The listing builds one solid part. Answer for the finished solid, in the listing's coordinates (mm). Face numbers are marked on the shaded views. A direction names the side the tool comes from. Coordinates: 2 decimals unless noted, no trailing zeros. Loops run counter-clockwise (first coordinate to the right, second up) from the corner with the lowest first, then second, coordinate; pieces in that order, holes last. Notation, with made-up numbers: (87, -23) - (109, -23) arc R32 cw to (109, 7) - close; hole circle Ø7 at (-29, 38.25). An arc over 180 degrees is marked (long way). Put each result on its own line as item: value.
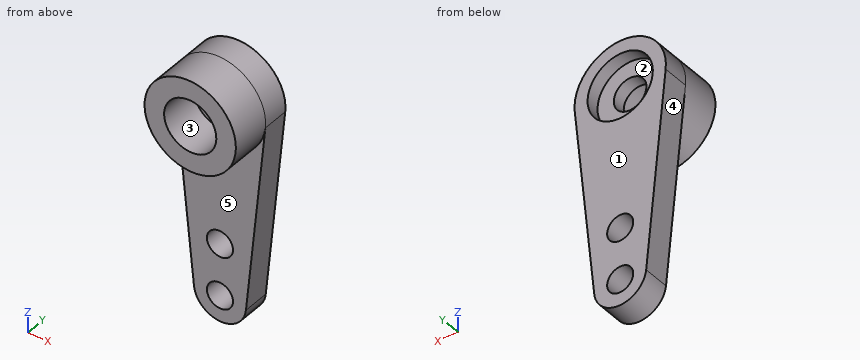
```python
from build123d import *

# Parameters (mm, degrees)
SKETCH_1_R          = 1
SKETCH_1_R_2        = 1.25
EXTRUDE_1_DEPTH     = 2
EXTRUDE_START       = 3
SKETCH_2_R          = 3.5
SKETCH_2_R_2        = 2
EXTRUDE_2_DEPTH     = 3
SKETCH_3_R          = 2.5
CUT_EXTRUDE_1_DEPTH = 1


with BuildPart() as part:
    # 草图1 → 凸台-拉伸1 (new body)
    with BuildSketch(Plane(origin=(0, 0, 0), x_dir=(1, 0, 0), z_dir=(0, 1, 0))):
        with BuildLine():
            Line((-3.48245603, 0.35), (-1.989974874, 15.2))
            ThreePointArc((-1.989974874, 15.2), (0, 17), (1.989974874, 15.2))
            Line((1.989974874, 15.2), (3.48245603, 0.35))
            ThreePointArc((3.48245603, 0.35), (0, -3.5), (-3.48245603, 0.35))
        make_face()
        with Locations(Location((0, 15, 0), (0, 0, 270))):
            Circle(SKETCH_1_R, mode=Mode.SUBTRACT)
        with Locations(Location((0, 11, 0), (0, 0, 270))):
            Circle(SKETCH_1_R, mode=Mode.SUBTRACT)
        with Locations(Location((0, 0, 0), (0, 0, 270))):
            Circle(SKETCH_1_R_2, mode=Mode.SUBTRACT)
    extrude(amount=EXTRUDE_1_DEPTH)

    # 草图2 → 凸台-拉伸2 (add)
    with BuildSketch(Plane.XZ.offset(EXTRUDE_START)):
        with Locations(Location((0, 0, 0), (0, 0, 270))):
            Circle(SKETCH_2_R)
        with Locations(Location((0, 0, 0), (0, 0, 270))):
            Circle(SKETCH_2_R_2, mode=Mode.SUBTRACT)
    extrude(amount=-EXTRUDE_2_DEPTH)

    # 草图3 → 切除-拉伸1 (cut)
    with BuildSketch(Plane(origin=(0, 2, 0), x_dir=(1, 0, 0), z_dir=(0, 1, 0))):
        with Locations(Location((0, 0, 0), (0, 0, 270))):
            Circle(SKETCH_3_R)
    extrude(amount=-CUT_EXTRUDE_1_DEPTH, mode=Mode.SUBTRACT)


solid = part.part
```
1) Straight lines are drawn through the part: L1, parallel to X at y = 0.45, z = 0; L2, parallel to Z at x = 0.5, y = 1.5; L3, parallel to Y at x = 2.25, z = -10.5. For each, find the intervals that lie inside material, in ascending order. Write a range as [from, to].
Found:
L1: x = [-3.5, -1.25], [1.25, 3.5]
L2: z = [-16.94, -15.87], [-14.13, -11.87], [-10.13, -2.45], [2.45, 3.46]
L3: y = [0, 2]
2) The part is cut by section A-A (z = 0). Give the vertices of the cut face in (x, y), and give its area (3 significant figures).
Found:
outline: (-3.5, -3) - (-2, -3) - (-2, 0) - (-1.25, 0) - (-1.25, 1) - (-2.5, 1) - (-2.5, 2) - (-3.5, 2) - close; (1.25, 0) - (2, 0) - (2, -3) - (3.5, -3) - (3.5, 2) - (2.5, 2) - (2.5, 1) - (1.25, 1) - close
area: 15.5 mm^2
3) The part is cut by section D-D (z = -15). Give the vertices of the cut face in (x, y).
Found:
outline: (-2.01, 0) - (-1, 0) - (-1, 2) - (-2.01, 2) - close; (1, 0) - (2.01, 0) - (2.01, 2) - (1, 2) - close
4) The part is cut by section B-B (x = 0). Give the vertices of the cut face in (y, z).
Found:
outline: (-3, -3.5) - (0, -3.5) - (0, -10) - (2, -10) - (2, -2.5) - (1, -2.5) - (1, -1.25) - (0, -1.25) - (0, -2) - (-3, -2) - close; (-3, 2) - (0, 2) - (0, 1.25) - (1, 1.25) - (1, 2.5) - (2, 2.5) - (2, 3.5) - (-3, 3.5) - close; (0, -17) - (2, -17) - (2, -16) - (0, -16) - close; (0, -14) - (2, -14) - (2, -12) - (0, -12) - close
5) Each of these flat-tipped pins is pushed along its axis until it touches: pin 1 (2 mm diameter, centred on x = 2.5, z = -8.5, fed in from -Y); pin 2 (2 mm diameter, centred on y = -2, z = -11.5, fed in from -X); pin 3 (3 mm diameter, centred on y = 0.5, z = -6, fed in from +X). Where does it stop, or does it pass through?
Found:
pin 1: stops at y = 0
pin 2: passes through
pin 3: stops at x = 3.07
6) For the marked faces 1 and 2, determine the directions among +Z, -Z, +X, -X, +Y, -Y from which every point of the face is accessible in a straight line to the end or side of a thin tool.
Found:
face 1: +Z, -Z, +X, -X, +Y
face 2: +Y
7) For a pull along Z with two mould halves and no side action, classify the marked faces 3, 4 and 5 as pulls with the +Z half, pulls with the -Z half, needs draft (parallel to the pull), parting line crosses it, or undercut.
Found:
face 3: undercut
face 4: pulls with the -Z half
face 5: needs draft
8) The part is cut by section C-C (y = 0.3). Give the vertices of the cut face in (x, z).
Found:
outline: (-3.48, -0.35) - (-1.99, -15.2) arc R2 ccw to (1.99, -15.2) - (3.48, -0.35) arc R3.5 ccw (long way) to start; hole circle Ø2.5 at (0, 0); hole circle Ø2 at (0, -15); hole circle Ø2 at (0, -11)
